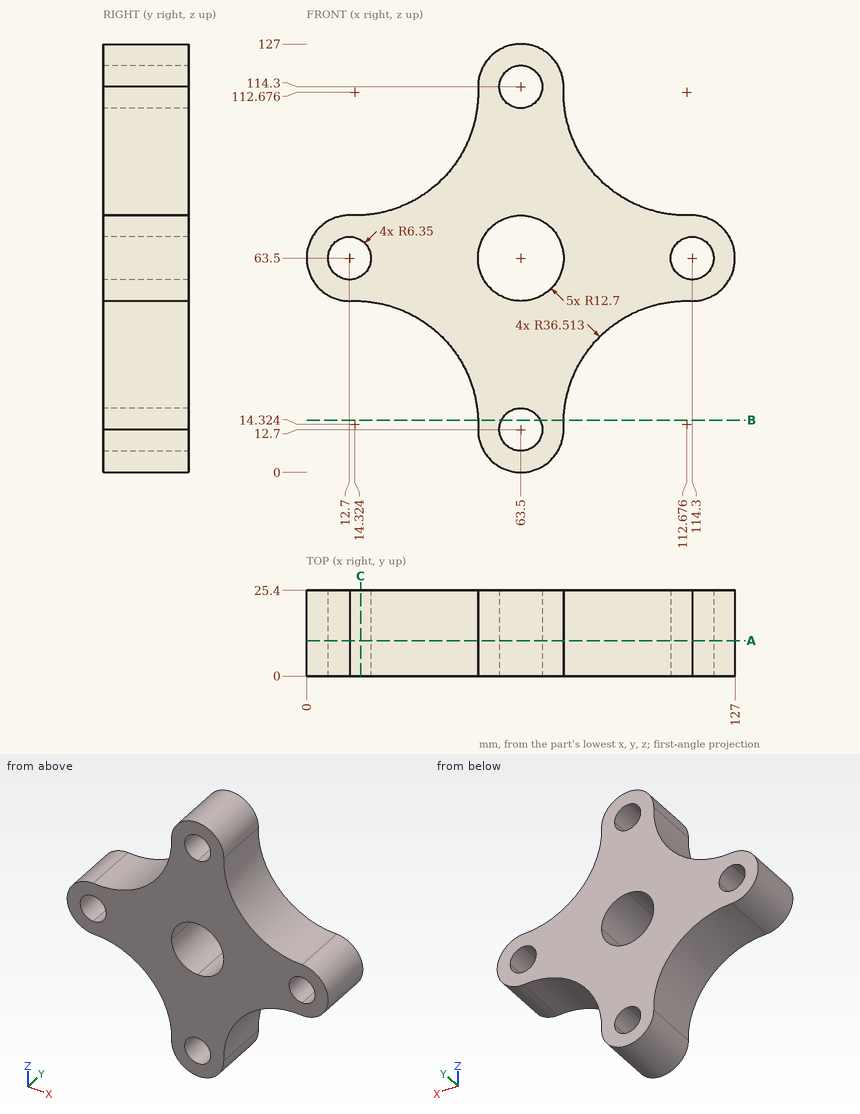
Input: dimensioned drawing with shaded views. Units: mm. Origin: part minimum x, y, z. Round coordinates to 2 decimals unless told otherwise and drop trailing zeros. Order: outer loops, then holes, each group sorted by start corner. A loop starts at its lowest first (then second) coordinate and runs counter-clockwise, first axis right, second up. Notation, with made-up numbers: (2.25, 67) -> (58.25, 67) arc R19 ccw to (58.25, 87) -> close; hole circle Ø6 at (-18, 15.5). An arc over 180 degrees is marked (long way). Put each result on its own line as item: value. Start each with the question number.
Q1. Section A-A on y = 10.5. Give the number of separate pieces and of enclosed holes in the cut face, and give its area (3 significant figures).
Q2. Section B-B on z = 15.5. Return the cut outline in (x, y).
Q3. Line query: probe 1 along X at (y, z) = (3, 60.5) (1 decimal); probe 2 along Z at (x, y) = (12, 22.5); probe 3 along Z at (x, y) = (67, 13.5). Output: solid intervals per line, ascending.
Q4. Section C-C on x = 16. Return the cut outline in (y, z) (1 decimal).
Q5. First-contact query: pin 1 (8 mm diameter, centred on y = 13.5, z = 107, fed in from +X); pin 2 (8 mm diameter, centred on x = 99, y = 5.5, fed in from -Z); pin 3 (10 mm diameter, centred on y = 15.5, z = 33.5, fed in from -X) (1 decimal); pin 4 (6 mm diameter, centred on x = 69.5, z = 105.5, fed in from -Y). Flat tips, straight axial feed; report the tip coordinate or a pass-through.
Ans:
1. separate pieces: 1
1. enclosed holes: 5
1. area: 5,650 mm2
2. outline: (50.82, 0) -> (57.8, 0) -> (57.8, 25.4) -> (50.82, 25.4) -> close; (69.2, 0) -> (76.18, 0) -> (76.18, 25.4) -> (69.2, 25.4) -> close
3. probe 1: x = 0.4 to 7.1, 18.3 to 51.2, 75.8 to 108.7, 119.9 to 126.6
3. probe 2: z = 50.82 to 57.19, 69.81 to 76.18
3. probe 3: z = 0.49 to 7.4, 18 to 51.29, 75.71 to 109, 119.6 to 126.51
4. outline: (0, 50.8) -> (25.4, 50.8) -> (25.4, 58.1) -> (0, 58.1) -> close; (0, 68.9) -> (25.4, 68.9) -> (25.4, 76.2) -> (0, 76.2) -> close
5. pin 1: stops at x = 77.47
5. pin 2: stops at z = 46.27
5. pin 3: stops at x = 41.7
5. pin 4: stops at y = 0
